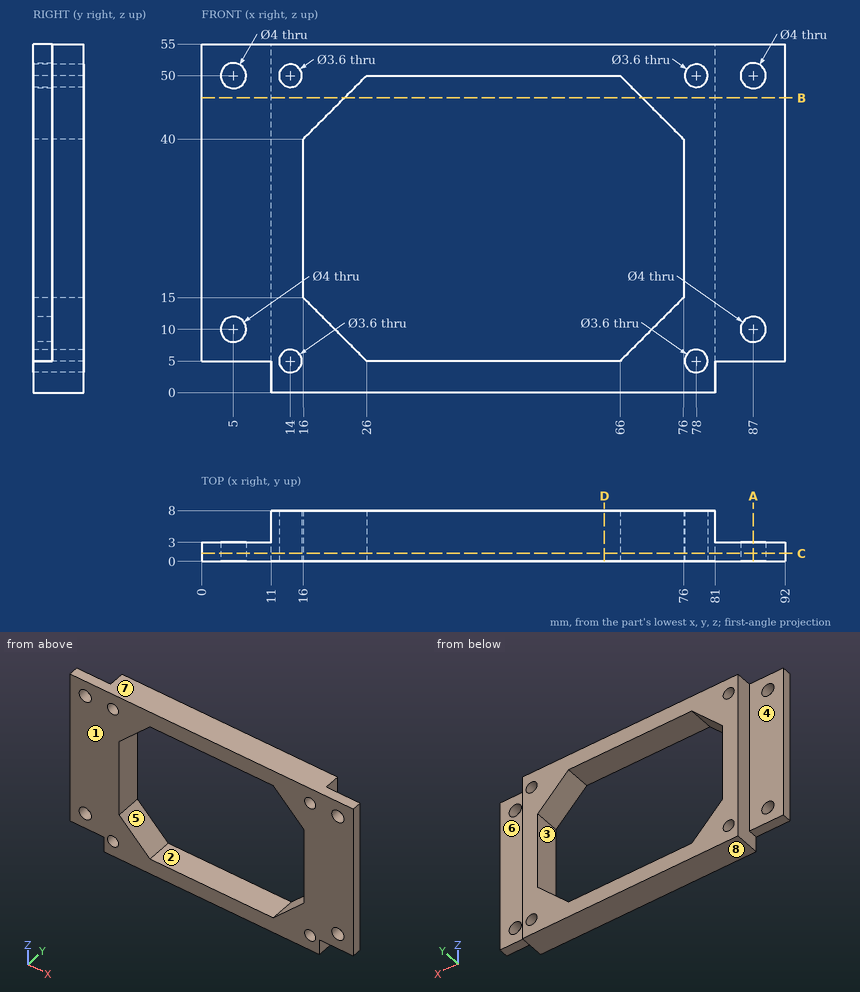
Design review of the part shown in the three views and the two pictorial views. Dimensions are in mm from the part's minimum x, y and z. A direction names the side the tool comes from. Round coordinates to 2 decimals unless told otherwise and drop trailing zeros. Write each loop counter-clockwise with the first axis right and the second up, starting at its lowest first coordinate (ties: lowest second). Pieces come first, ordered by that corner, then holes.
1) Take a section at C-C on y = 1.25. State how many separate pieces and enclosed holes the cut face has, then the cut area to 3 significant figures.
Answer below:
separate pieces: 1
enclosed holes: 9
area: 2,360 mm2
2) Take a section at A-A on x = 87. Give the boundary of the cut face in (y, z).
Answer below:
outline: (0, 5) - (3, 5) - (3, 8) - (0, 8) - close; (0, 12) - (3, 12) - (3, 48) - (0, 48) - close; (0, 52) - (3, 52) - (3, 55) - (0, 55) - close
3) Mouldability with a two-part tool opening along X and no side actions: class the marked faces 1, 2 and 3 as +X half, -X half, draft (parallel to the pull), parting line (faces both ways), or undercut.
Answer below:
face 1: draft
face 2: undercut
face 3: undercut
4) For line 1 along Z through (x, y) = (87, 2.2); line 2 along Z through (x, y) = (39, 5); line 3 along X through (y, z) = (1, 25), list the stretches that pass through material, from the lowest coordinate up.
Answer below:
line 1: z = 5 to 8, 12 to 48, 52 to 55
line 2: z = 0 to 5, 50 to 55
line 3: x = 0 to 16, 76 to 92
5) Take a section at B-B on z = 46.5. Give the boundary of the cut face in (x, y), then the cut area to 3 significant figures.
Answer below:
outline: (0, 0) - (22.5, 0) - (22.5, 8) - (11, 8) - (11, 3) - (0, 3) - close; (69.5, 0) - (92, 0) - (92, 3) - (81, 3) - (81, 8) - (69.5, 8) - close
area: 250 mm2
6) Insertion check: pin 1 Ø2.5 at (y, z) = (4, 33.5) entering from +X; pin 2 Ø1.5 at (x, y) = (8, 1) entering from -Z; pin 3 Ø3 at (x, z) = (78, 50) entering from -Y; pin 4 Ø9 at (x, z) = (3, 34.5) entering from +Y. Each pin has a flat end and moves straight along its axis. Give the tip position at first contact, or say it passes through.
Answer below:
pin 1: stops at x = 92
pin 2: stops at z = 5
pin 3: passes through
pin 4: stops at y = 3
7) Machinability: for the marked faces 4, 5, 6, 7 and 8, which of the approach directions +Z, -Z, +X, -X, +Y, -Y give a long, thin tool a straight path to every point of the face, cutting with its end or side? Answer none if there is none.
Answer below:
face 4: +Z, -Z, -X, +Y
face 5: +Y, -Y
face 6: +Z, -Z, +X, +Y
face 7: +Z, +X, -X, +Y, -Y
face 8: -Z, +X, -X, +Y, -Y
8) Take a section at D-D on x = 63.5. Give the boundary of the cut face in (y, z).
Answer below:
outline: (0, 0) - (8, 0) - (8, 5) - (0, 5) - close; (0, 50) - (8, 50) - (8, 55) - (0, 55) - close
